Build history of the part. All positions in model axes, mm. A direction names the side the tool comes from. Round coordinates to 2 decimals unless told otherwise and drop trailing zeros. Write each loop counter-clockwise with the first axis right and the second up, starting at its lowest first coordinate (ties: lowest second). Pieces come first, ordered by that corner, then holes. Notation, with made-up numbers: (-1, 23.5) -> (23, 23.5) arc R19 ccw to (23, 54.5) -> close; hole circle Ø8 at (66, 64.5). An arc over 180 degrees is marked (long way). One line per question, with ' | ' between items.
Autodesk Inventor part; units mm, degrees
ref_plane "YZ Plane" through (0, 0, 0) normal (1, 0, 0) x (0, 1, 0)
ref_plane "XZ Plane" through (0, 0, 0) normal (0, 1, 0) x (-1, 0, 0)
ref_plane "XY Plane" through (0, 0, 0) normal (0, 0, 1) x (1, 0, 0)
sketch "Sketch1" plane through (0, 0, 0) normal (0, 0, 1) x (1, 0, 0)
  line L0 (0, 0) -> (63, 0)
  line L1 (53.5, -25.4) -> (41.5, -25.4)
  line L2 (41.5, -25.4) -> (41.5, -12.5)
  line L3 (41.5, -12.5) -> (21.5, -12.5)
  line L4 (21.5, -12.5) -> (21.5, -25.4)
  line L5 (0, 0) -> (0, -8.9)
  line L6 (0, -8.9) -> (5, -8.9)
  line L7 (5, -8.9) -> (9.5, -25.4)
  line L8 (9.5, -25.4) -> (21.5, -25.4)
  line L9 (53.5, -25.4) -> (58, -8.9)
  line L10 (58, -8.9) -> (63, -8.9)
  line L11 (63, -8.9) -> (63, 0)
  point P0 (31.5, -12.5)
  point P1 (31.5, 0)
  dimension "d0" = 63
  dimension "d1" = 25.4
  dimension "d4" = 21.5
  dimension "d5" = 8.9
  dimension "d6" = 12.9
  dimension "d7" = 12
  dimension "d8" = 5
extrude "Extrusion1" add sketch "Sketch1" along normal blind 50.5
sketch "Sketch2" plane through (0, 0, 50.5) normal (0, 0, 1) x (1, 0, 0)
  line L0 (21.5, -25.4) -> (21.5, -12.5)
  line L1 (41.5, -12.5) -> (41.5, -25.4)
  line L2 (9.5, -25.4) -> (21.5, -25.4)
  line L3 (41.5, -25.4) -> (53.5, -25.4)
  line L4 (9.5, -25.4) -> (9.5, 0)
  line L5 (9.5, 0) -> (53.5, 0)
  line L6 (53.5, 0) -> (53.5, -25.4)
  line L7 (21.5, -12.5) -> (41.5, -12.5)
  point P0 (0, 0)
  point P1 (31.5, 0)
extrude "Extrusion2" add sketch "Sketch2" along normal blind 13.5 and the other way blind 64
sketch "Sketch3" plane through (63, 0, 50.5) normal (0, 1, 0) x (1, 0, 0)
  circle A0 centre (-58, 5.25) radius 3
  circle A1 centre (-58, 45.25) radius 3
  circle A2 centre (-5, 5.25) radius 3
  circle A3 centre (-5, 45.25) radius 3
  line L0 (-58, 5.25) -> (-5, 5.25) construction
  line L1 (-5, 5.25) -> (-5, 45.25) construction
  line L2 (-5, 45.25) -> (-58, 45.25) construction
  line L3 (-58, 45.25) -> (-58, 5.25) construction
  line L4 (-53.5, 64) -> (-9.5, 64)
  line L5 (-63, 50.5) -> (-63, 0)
  point P0 (-31.5, 64)
  point P1 (-31.5, 45.25)
  point P2 (-58, 25.25)
  point P3 (-63, 25.25)
  dimension "d15" = 6
  dimension "d16" = 40
  dimension "d17" = 53
extrude "Extrusion3" cut sketch "Sketch3" against normal blind 34.5
properties part number "HGW20CC_Slider"
(1) Slice it at D-D (x = 6.5). Write the cut outline in (y, z), then the cut area to 3 significant figures.
Calculated:
outline: (-14.4, 0) -> (0, 0) -> (0, 2.65) -> (-14.4, 2.65) -> close; (-14.4, 7.85) -> (0, 7.85) -> (0, 42.65) -> (-14.4, 42.65) -> close; (-14.4, 47.85) -> (0, 47.85) -> (0, 50.5) -> (-14.4, 50.5) -> close | area: 578 mm2
(2) Drop flat-ended pins along their axis: pin 1 (5 mm diameter, centred on x = 56.5, y = -14.5, fed in from -Z); pin 2 (4 mm diameter, centred on y = -8.5, z = -9.5, fed in from -X); pin 3 (3 mm diameter, centred on y = -17, z = 46, fed in from -X); pin 4 (3.5 mm diameter, centred on x = 5, z = 5.25, fed in from +Y). Give the stop position or say it passes through.
Calculated:
pin 1: z = 0 | pin 2: x = 9.5 | pin 3: x = 7.07 | pin 4: through
(3) Mould opens along X. For faces 1 (the cylindrical face through (55.003, -7.614, 5.118)), 2 (the flat face through (7.219, -17.034, 24.896)), 3 (the flat face through (31, -10, 64)) say: pulls with the +X half, pulls with the -X half, needs draft (parallel to the pull), parting line crosses it, or undercut.
Calculated:
face 1: undercut | face 2: pulls with the -X half | face 3: needs draft
(4) Slice it at C-C (y = -17.75). Write the cut outline in (x, z), then the cut area to 3 significant figures.
Calculated:
outline: (7.41, 0) -> (9.5, 0) -> (9.5, -13.5) -> (21.5, -13.5) -> (21.5, 64) -> (9.5, 64) -> (9.5, 50.5) -> (7.41, 50.5) -> (7.41, 47.03) arc R3 cw to (7.41, 43.47) -> (7.41, 7.03) arc R3 cw to (7.41, 3.47) -> close; (41.5, -13.5) -> (53.5, -13.5) -> (53.5, 0) -> (55.59, 0) -> (55.59, 3.47) arc R3 cw to (55.59, 7.03) -> (55.59, 43.47) arc R3 cw to (55.59, 47.03) -> (55.59, 50.5) -> (53.5, 50.5) -> (53.5, 64) -> (41.5, 64) -> close | area: 2,070 mm2
(5) Wall check: line 1 (Z direction, x = 58, y = -6.25); line 2 (X direction, y = -21, z = 56); line 3 (X direction, y = -8.75, z = 7). Give the ranges that are in metal, low to high. Write a range as from..to.
Calculated:
line 1: 0..2.25, 8.25..42.25, 48.25..50.5 | line 2: 9.5..21.5, 41.5..53.5 | line 3: 0..2.56, 7.44..55.56, 60.44..63
(6) Slice it at A-A (z = 5.25). Write the cut outline in (x, y), then the cut area to 3 significant figures.
Calculated:
outline: (0, -8.9) -> (2, -8.9) -> (2, 0) -> (0, 0) -> close; (8, -19.9) -> (9.5, -25.4) -> (21.5, -25.4) -> (21.5, -12.5) -> (41.5, -12.5) -> (41.5, -25.4) -> (53.5, -25.4) -> (55, -19.9) -> (55, 0) -> (8, 0) -> close; (61, -8.9) -> (63, -8.9) -> (63, 0) -> (61, 0) -> close | area: 963 mm2
(7) Slice it at B-B (z = 58.5). Write the cut outline in (x, y).
Calculated:
outline: (9.5, -25.4) -> (21.5, -25.4) -> (21.5, -12.5) -> (41.5, -12.5) -> (41.5, -25.4) -> (53.5, -25.4) -> (53.5, 0) -> (9.5, 0) -> close
(8) 3-axis set-ups, long thin cutter, end or side, ignore diameter. For faces 4 (the flat face through (57, -7, 0)), 5 (the flat face through (6, -7, 0)), 6 (the flat face through (6, -7, 50.5)): which of +Z, -Z, +X, -X, +Y, -Y reach the whole face in a straight line?
Calculated:
face 4: -Z, +X, +Y, -Y | face 5: -Z, -X, +Y, -Y | face 6: +Z, -X, +Y, -Y
